```python
from build123d import *

# Parameters (mm, degrees)
SKETCH1_W               = 40
SKETCH1_H               = 64
BOSS_EXTRUDE1_DEPTH     = 1
SKETCH2_W               = 20
SKETCH2_H               = 33
SKETCH2_R               = 1.5
CUT_EXTRUDE1_DEPTH      = 1
CUT_EXTRUDE1_DEPTH_BACK = 2


with BuildPart() as part:
    # Sketch1 → Boss-Extrude1 (new body)
    with BuildSketch(Plane.XY):
        with Locations((20, 5.82585752)):
            Rectangle(SKETCH1_W, SKETCH1_H)
    extrude(amount=BOSS_EXTRUDE1_DEPTH)

    # Sketch2 → Cut-Extrude1 (cut, two sides)
    with BuildSketch(Plane.XY.offset(1)) as cut_extrude1_sk:
        with Locations((20, 5.82585752)):
            Rectangle(SKETCH2_W, SKETCH2_H)
        with Locations((4, -19.67414248)):
            Circle(SKETCH2_R)
        with Locations((4, -2.67414248)):
            Circle(SKETCH2_R)
        with Locations((4, 14.32585752)):
            Circle(SKETCH2_R)
        with Locations((4, 31.32585752)):
            Circle(SKETCH2_R)
        with Locations((36, -19.67414248)):
            Circle(SKETCH2_R)
        with Locations((36, -2.67414248)):
            Circle(SKETCH2_R)
        with Locations((36, 14.32585752)):
            Circle(SKETCH2_R)
        with Locations((36, 31.32585752)):
            Circle(SKETCH2_R)
    extrude(amount=CUT_EXTRUDE1_DEPTH, mode=Mode.SUBTRACT)
    extrude(cut_extrude1_sk.sketch, amount=-CUT_EXTRUDE1_DEPTH_BACK, mode=Mode.SUBTRACT)


solid = part.part
```
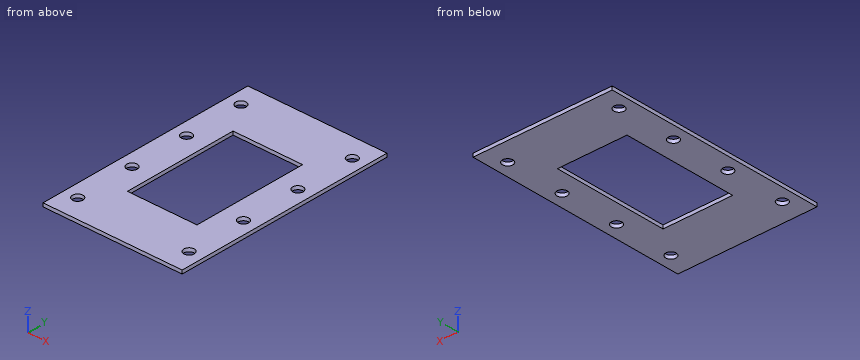
Model file for the job. Use its own axes, mm. Give positions to 0.01 mm unless a question says otherwise; leave off trailing zeros. Order: outer loops, then holes, each group sorted by start corner. A loop starts at its lowest first (then second) coordinate and runs counter-clockwise, first axis right, second up.
1) Saw through at A-A, the plane y = 5.5. Write the cut outline in (x, z), then the cut area to 3 significant figures.
2) Saw through at C-C, the plane y = -2. Write the cut outline in (x, z), then the cut area to 3 significant figures.
3) Saw through at D-D, the plane x = 4. Write the cut outline in (y, z), then the cut area to 3 significant figures.
4) Wall check: probe 1 along Y at (x, z) = (36, 0.3); probe 2 along Y at (x, z) = (23.5, 0.2); probe 3 along Y at (x, z) = (36.5, 0.85). Give the ranges that are in metal, low to high.
5) Saw through at B-B, the plane x = 11.5. Write the cut outline in (y, z).
Computed:
1. outline: (0, 0) - (10, 0) - (10, 1) - (0, 1) - close; (30, 0) - (40, 0) - (40, 1) - (30, 1) - close
1. area: 20.0 mm2
2. outline: (0, 0) - (2.66, 0) - (2.66, 1) - (0, 1) - close; (5.34, 0) - (10, 0) - (10, 1) - (5.34, 1) - close; (30, 0) - (34.66, 0) - (34.66, 1) - (30, 1) - close; (37.34, 0) - (40, 0) - (40, 1) - (37.34, 1) - close
2. area: 14.6 mm2
3. outline: (-26.17, 0) - (-21.17, 0) - (-21.17, 1) - (-26.17, 1) - close; (-18.17, 0) - (-4.17, 0) - (-4.17, 1) - (-18.17, 1) - close; (-1.17, 0) - (12.83, 0) - (12.83, 1) - (-1.17, 1) - close; (15.83, 0) - (29.83, 0) - (29.83, 1) - (15.83, 1) - close; (32.83, 0) - (37.83, 0) - (37.83, 1) - (32.83, 1) - close
3. area: 52.0 mm2
4. probe 1: y = -26.17 to -21.17, -18.17 to -4.17, -1.17 to 12.83, 15.83 to 29.83, 32.83 to 37.83
4. probe 2: y = -26.17 to -10.67, 22.33 to 37.83
4. probe 3: y = -26.17 to -21.09, -18.26 to -4.09, -1.26 to 12.91, 15.74 to 29.91, 32.74 to 37.83
5. outline: (-26.17, 0) - (-10.67, 0) - (-10.67, 1) - (-26.17, 1) - close; (22.33, 0) - (37.83, 0) - (37.83, 1) - (22.33, 1) - close
